Can you work these out from the model? Positions are in its coordinate system, mm. Face numbers are marked on the shaded views. A direction names the side the tool comes from. Round coordinates to 2 decimals unless told otherwise and drop trailing zeros. Write each loop counter-clockwise with the first axis right and the second up, starting at its lowest first coordinate (ties: lowest second). Pieces come first, ordered by that corner, then holes. Notation, with made-up numbers: M -37.75,6 L 20.25,6 A7 ccw 20.25,16 Z; hole C -36,70.5 d2. An arc over 180 degrees is marked long. Answer in a Markdown table with one row per item. Add a question column.
(1) I'm going to push flat-ended pins straight in: pin 1 (6.5 mm diameter, centred on y = 5, z = -67.5, fed in from -X); pin 2 (8 mm diameter, centred on x = 75, z = -43.5, fed in from -Y); pin 3 (1.8 mm diameter, centred on y = 98.5, z = -7, fed in from +X). Where does each tip first touch, or does it pass through?
(2) Suppose I cut it at C-C, the plane z = -55.5. Write out the boundary of the cut face in (x, y).
(3) For the marked faces 1 and 2, which set-ups out of +Z, -Z, +X, -X, +Y, -Y let a thin tool reach every point of the face, with its end or its side?
(4) Suppose I cut it at A-A, the plane x = 0. Count the separate pieces of the cut face and the enclosed holes in it, then the cut area to 3 significant figures.
(5) If I drill on probe 1 along X at (y, z) = (72, 10); probe 2 along Z at (x, y) = (69, 81); probe 3 along Z at (x, y) = (-67.5, 1.5), over which ranges is the centre line in solid material (lowest first)?
(6) If we mould it in two halves opening along X, with no side actions, what happens to the marked faces 3, 4, 5 and 6? For each: released by +X, released by -X, zero draft, split by the parting line, or undercut.
(7) Suppose I cut it at D-D, the plane z = 12.5. Write out the boundary of the cut face in (x, y).
(8) Suppose I cut it at B-B, the plane y = 15. Write out the boundary of the cut face in (x, z), then the cut area to 3 significant figures.
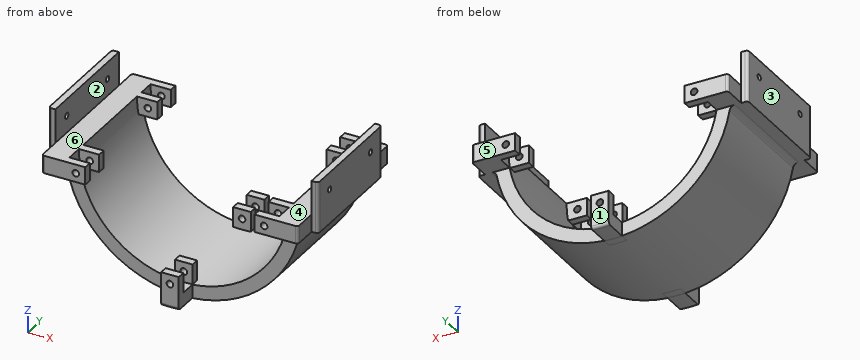
from build123d import *
from build123d.topology import SkipClean

# Parameters (mm, degrees)
BOSS_EXTRUDE1_DEPTH  = 84.17
BOSS_EXTRUDE2_START  = -0.5
SKETCH3_W            = 32
SKETCH3_H            = 13
BOSS_EXTRUDE2_DEPTH  = 6
BOSS_EXTRUDE3_DEPTH  = 11.5
SKETCH5_W            = 32
SKETCH5_H            = 13
BOSS_EXTRUDE4_DEPTH  = 6
SKETCH7_R            = 2.15
CUT_EXTRUDE1_DEPTH   = 240.98758072
BOSS_EXTRUDE5_START  = -0.5
SKETCH9_W            = 30.514448454
SKETCH9_H            = 13
BOSS_EXTRUDE5_DEPTH  = 6
BOSS_EXTRUDE6_START  = 12
BOSS_EXTRUDE6_DEPTH  = 12
SKETCH12_W           = 32
SKETCH12_H           = 13
BOSS_EXTRUDE7_DEPTH  = 6
SKETCH14_R           = 2.45
CUT_EXTRUDE2_DEPTH   = 179.542456856
BOSS_EXTRUDE8_START  = -6.5
BOSS_EXTRUDE8_DEPTH  = 6
BOSS_EXTRUDE9_DEPTH  = 11.5
BOSS_EXTRUDE10_DEPTH = 6
BOSS_EXTRUDE11_START = -0.5
BOSS_EXTRUDE11_DEPTH = 6
BOSS_EXTRUDE12_START = 12
BOSS_EXTRUDE12_DEPTH = 12
BOSS_EXTRUDE13_START = 6
BOSS_EXTRUDE13_DEPTH = 6
SKETCH19_R           = 2.45
CUT_EXTRUDE3_DEPTH   = 179.542456856
FILLET4_R            = 2
FILLET5_R            = 4


with BuildPart() as part:
    # Sketch1 → Boss-Extrude1 (new body)
    with BuildSketch(Plane(origin=(0, 0, 0), x_dir=(1, 0, 0), z_dir=(0, 1, 0))):
        with BuildLine():
            Line((-86.528896907, 13), (-99.5, 13))
            Line((-99.5, 13), (-99.5, -25))
            Line((-99.5, -25), (-94.5, -25))
            Line((-94.5, -25), (-94.5, 0))
            Line((-94.5, 0), (-77.5, 0))
            ThreePointArc((-77.5, 0), (0, 77.5), (77.5, 0))
            Line((77.5, 0), (94.5, 0))
            Line((94.5, 0), (94.5, -25))
            Line((94.5, -25), (99.5, -25))
            Line((99.5, -25), (99.5, 13))
            Line((99.5, 13), (86.528896907, 13))
            ThreePointArc((86.528896907, 13), (0, 87.5), (-86.528896907, 13))
        make_face()
    extrude(amount=BOSS_EXTRUDE1_DEPTH)

    # Sketch3 → Boss-Extrude2 (add)
    with BuildSketch(Plane(origin=(0, 84.17, 0), x_dir=(1, 0, 0), z_dir=(0, 1, 0)).offset(BOSS_EXTRUDE2_START)):
        with Locations((-78.5, 6.5)):
            Rectangle(SKETCH3_W, SKETCH3_H)
        with Locations((78.5, 6.5)):
            Rectangle(SKETCH3_W, SKETCH3_H)
    extrude(amount=-BOSS_EXTRUDE2_DEPTH)

    # Sketch4 → Boss-Extrude3 (add)
    with SkipClean():  # the faces are left unmerged after this step: merging them gives an invalid solid
        with BuildSketch(Plane(origin=(0, 84.17, 0), x_dir=(1, 0, 0), z_dir=(0, 1, 0))):
            with BuildLine():
                Line((-94.5, 13), (-76.401897882, 13))
                ThreePointArc((-76.401897882, 13), (-77.224986519, 6.523147788), (-77.5, 0))
                Line((-77.5, 0), (-94.5, 0))
                Line((-94.5, 0), (-94.5, 13))
            make_face()
            with BuildLine():
                Line((76.401897882, 13), (94.5, 13))
                Line((94.5, 13), (94.5, 0))
                Line((94.5, 0), (77.5, 0))
                ThreePointArc((77.5, 0), (77.224986519, 6.523147788), (76.401897882, 13))
            make_face()
        extrude(amount=BOSS_EXTRUDE3_DEPTH)

    # Sketch5 → Boss-Extrude4 (add)
    with SkipClean():  # the faces are left unmerged after this step: merging them gives an invalid solid
        with BuildSketch(Plane(origin=(0, 95.67, 0), x_dir=(1, 0, 0), z_dir=(0, 1, 0))):
            with Locations((-78.5, 6.5)):
                Rectangle(SKETCH5_W, SKETCH5_H)
            with Locations((78.5, 6.5)):
                Rectangle(SKETCH5_W, SKETCH5_H)
        extrude(amount=BOSS_EXTRUDE4_DEPTH)

    # Sketch7 → Cut-Extrude1 (cut, through all)
    with SkipClean():  # the faces are left unmerged after this step: merging them gives an invalid solid
        with BuildSketch(Plane.ZY.offset(99.5)):
            with Locations((12.5, 69.17)):
                Circle(SKETCH7_R)
            with Locations((12.5, 15)):
                Circle(SKETCH7_R)
        extrude(amount=-CUT_EXTRUDE1_DEPTH, mode=Mode.SUBTRACT)

    # Sketch9 → Boss-Extrude5 (add)
    with SkipClean():  # the faces are left unmerged after this step: merging them gives an invalid solid
        with BuildSketch(Plane.XZ.offset(BOSS_EXTRUDE5_START)):
            with Locations((-77.757224227, -6.5)):
                Rectangle(SKETCH9_W, SKETCH9_H)
            with Locations((77.757224227, -6.5)):
                Rectangle(SKETCH9_W, SKETCH9_H)
        extrude(amount=-BOSS_EXTRUDE5_DEPTH)

    # Sketch11 → Boss-Extrude6 (add)
    with SkipClean():  # the faces are left unmerged after this step: merging them gives an invalid solid
        with BuildSketch(Plane.XZ.offset(BOSS_EXTRUDE6_START)):
            with BuildLine():
                Line((-94.5, 0), (-77.5, 0))
                ThreePointArc((-77.5, 0), (-77.224986519, -6.523147788), (-76.401897882, -13))
                Line((-76.401897882, -13), (-94.5, -13))
                Line((-94.5, -13), (-94.5, 0))
            make_face()
            with BuildLine():
                Line((94.5, 0), (77.5, 0))
                ThreePointArc((77.5, 0), (77.224986519, -6.523147788), (76.401897882, -13))
                Line((76.401897882, -13), (94.5, -13))
                Line((94.5, -13), (94.5, 0))
            make_face()
        extrude(amount=-BOSS_EXTRUDE6_DEPTH)

    # Sketch12 → Boss-Extrude7 (add)
    with SkipClean():  # the faces are left unmerged after this step: merging them gives an invalid solid
        with BuildSketch(Plane.XZ.offset(12)):
            with Locations((-78.5, -6.5)):
                Rectangle(SKETCH12_W, SKETCH12_H)
            with Locations((78.5, -6.5)):
                Rectangle(SKETCH12_W, SKETCH12_H)
        extrude(amount=BOSS_EXTRUDE7_DEPTH)

    # Sketch14 → Cut-Extrude2 (cut, through all)
    with SkipClean():  # the faces are left unmerged after this step: merging them gives an invalid solid
        with BuildSketch(Plane(origin=(0, 101.67, 0), x_dir=(1, 0, 0), z_dir=(0, 1, 0))):
            with Locations(Location((-69.5, 6.5, 0), (0, 0, 270))):
                Circle(SKETCH14_R)
            with Locations(Location((69.5, 6.5, 0), (0, 0, 270))):
                Circle(SKETCH14_R)
        extrude(amount=-CUT_EXTRUDE2_DEPTH, mode=Mode.SUBTRACT)

    # Sketch15 → Boss-Extrude8 (add)
    with SkipClean():  # the faces are left unmerged after this step: merging them gives an invalid solid
        with BuildSketch(Plane(origin=(0, 84.17, 0), x_dir=(1, 0, 0), z_dir=(0, 1, 0)).offset(BOSS_EXTRUDE8_START)):
            with BuildLine():
                Line((-6.5, 87.258237433), (-6.5, 62.5))
                Line((-6.5, 62.5), (6.5, 62.5))
                Line((6.5, 62.5), (6.5, 87.258237433))
                ThreePointArc((6.5, 87.258237433), (0, 87.5), (-6.5, 87.258237433))
            make_face()
        extrude(amount=BOSS_EXTRUDE8_DEPTH)

    # Sketch17 → Boss-Extrude9 (add)
    with SkipClean():  # the faces are left unmerged after this step: merging them gives an invalid solid
        with BuildSketch(Plane(origin=(0, 84.17, 0), x_dir=(1, 0, 0), z_dir=(0, 1, 0))):
            with BuildLine():
                Line((-6.5, 77.226938305), (-6.5, 87.258237433))
                ThreePointArc((-6.5, 87.258237433), (0, 87.5), (6.5, 87.258237433))
                Line((6.5, 87.258237433), (6.5, 77.226938305))
                ThreePointArc((6.5, 77.226938305), (0, 77.5), (-6.5, 77.226938305))
            make_face()
        extrude(amount=BOSS_EXTRUDE9_DEPTH)

    # Sketch18 → Boss-Extrude10 (add)
    with SkipClean():  # the faces are left unmerged after this step: merging them gives an invalid solid
        with BuildSketch(Plane(origin=(0, 95.67, 0), x_dir=(1, 0, 0), z_dir=(0, 1, 0))):
            with BuildLine():
                Line((-6.5, 87.258237433), (-6.5, 62.5))
                Line((-6.5, 62.5), (6.5, 62.5))
                Line((6.5, 62.5), (6.5, 87.258237433))
                ThreePointArc((6.5, 87.258237433), (0, 87.5), (-6.5, 87.258237433))
            make_face()
        extrude(amount=BOSS_EXTRUDE10_DEPTH)

    # Sketch20 → Boss-Extrude11 (add)
    with SkipClean():  # the faces are left unmerged after this step: merging them gives an invalid solid
        with BuildSketch(Plane.XZ.offset(BOSS_EXTRUDE11_START)):
            with BuildLine():
                Line((-6.5, -62.5), (6.5, -62.5))
                Line((6.5, -62.5), (6.5, -87.258237433))
                ThreePointArc((6.5, -87.258237433), (0, -87.5), (-6.5, -87.258237433))
                Line((-6.5, -87.258237433), (-6.5, -62.5))
            make_face()
        extrude(amount=-BOSS_EXTRUDE11_DEPTH)

    # Sketch21 → Boss-Extrude12 (add)
    with SkipClean():  # the faces are left unmerged after this step: merging them gives an invalid solid
        with BuildSketch(Plane.XZ.offset(BOSS_EXTRUDE12_START)):
            with BuildLine():
                Line((-6.5, -77.226938305), (-6.5, -87.258237433))
                ThreePointArc((-6.5, -87.258237433), (0, -87.5), (6.5, -87.258237433))
                Line((6.5, -87.258237433), (6.5, -77.226938305))
                ThreePointArc((6.5, -77.226938305), (0, -77.5), (-6.5, -77.226938305))
            make_face()
        extrude(amount=-BOSS_EXTRUDE12_DEPTH)

    # Sketch22 → Boss-Extrude13 (add)
    with SkipClean():  # the faces are left unmerged after this step: merging them gives an invalid solid
        with BuildSketch(Plane.XZ.offset(12).offset(BOSS_EXTRUDE13_START)):
            with BuildLine():
                Line((-6.5, -87.258237433), (-6.5, -62.5))
                Line((-6.5, -62.5), (6.5, -62.5))
                Line((6.5, -62.5), (6.5, -87.258237433))
                ThreePointArc((6.5, -87.258237433), (0, -87.5), (-6.5, -87.258237433))
            make_face()
        extrude(amount=-BOSS_EXTRUDE13_DEPTH)

    # Sketch19 → Cut-Extrude3 (cut, through all)
    with SkipClean():  # the faces are left unmerged after this step: merging them gives an invalid solid
        with BuildSketch(Plane(origin=(0, 101.67, 0), x_dir=(1, 0, 0), z_dir=(0, 1, 0))):
            with Locations(Location((0, 69.5, 0), (0, 0, 270))):
                Circle(SKETCH19_R)
        extrude(amount=-CUT_EXTRUDE3_DEPTH, mode=Mode.SUBTRACT)

    # Fillet4
    fillet4_edges = [part.edges().sort_by_distance(p)[0] for p in [
        (-94.5, 101.67, -6.5),
        (99.5, 0, 6),
        (94.5, 101.67, -6.5),
        (-99.5, 84.17, 6),
        (-99.5, 0, 6),
        (-94.5, -18, -6.5),
        (94.5, -18, -6.5),
        (0, 101.67, -87.5),
        (0, -18, -87.5),
        (99.5, 84.17, 6),
    ]]
    fillet(fillet4_edges, radius=FILLET4_R)

    # Fillet5
    fillet5_edges = [part.edges().sort_by_distance(p)[0] for p in [
        (86.528896907, 42.085, -13),
        (-86.528896907, 42.085, -13),
    ]]
    fillet(fillet5_edges, radius=FILLET5_R)


solid = part.part
Calculated:
| question | item | result |
|---|---|---|
| 1 | pin 1 | x = -59.4 |
| 1 | pin 2 | y = 0 |
| 1 | pin 3 | x = 94.5 |
| 2 | outline | M -67.65,0 L -54.09,0 L -54.09,84.17 L -67.65,84.17 Z; M 54.09,0 L 67.65,0 L 67.65,84.17 L 54.09,84.17 Z |
| 3 | face 1 | +Z, -Z, +X, -X, +Y |
| 3 | face 2 | +Z, +Y, -Y |
| 4 | separate pieces | 5 |
| 4 | enclosed holes | 0 |
| 4 | area | 1,440 mm² |
| 5 | probe 1 | -99.5 to -94.5, 94.5 to 99.5 |
| 5 | probe 2 | -53.81 to -35.29, -13 to -8.9, -4.1 to 0 |
| 5 | probe 3 | -55.68 to -38.08, -13 to -7.92, -5.08 to 0 |
| 6 | face 3 | released by -X |
| 6 | face 4 | undercut |
| 6 | face 5 | zero draft |
| 6 | face 6 | undercut |
| 7 | outline | M -99.5,2 A2 ccw -97.5,0 L -94.5,0 L -94.5,12.85 L -99.5,12.85 Z; M -99.5,17.15 L -94.5,17.15 L -94.5,67.02 L -99.5,67.02 Z; M -99.5,71.32 L -94.5,71.32 L -94.5,84.17 L -97.5,84.17 A2 ccw -99.5,82.17 Z; M 94.5,0 L 97.5,0 A2 ccw 99.5,2 L 99.5,12.85 L 94.5,12.85 Z; M 94.5,17.15 L 99.5,17.15 L 99.5,67.02 L 94.5,67.02 Z; M 94.5,71.32 L 99.5,71.32 L 99.5,82.17 A2 ccw 97.5,84.17 L 94.5,84.17 Z |
| 8 | outline | M -99.5,-13 L -89.91,-13 A4 cw -85.98,-16.26 A87.5 ccw 85.98,-16.26 A4 cw 89.91,-13 L 99.5,-13 L 99.5,10.35 L 94.5,10.35 L 94.5,0 L 77.5,0 A77.5 cw -77.5,0 L -94.5,0 L -94.5,10.35 L -99.5,10.35 Z; M -99.5,14.65 L -94.5,14.65 L -94.5,25 L -99.5,25 Z; M 94.5,14.65 L 99.5,14.65 L 99.5,25 L 94.5,25 Z |
| 8 | area | 3,120 mm² |
